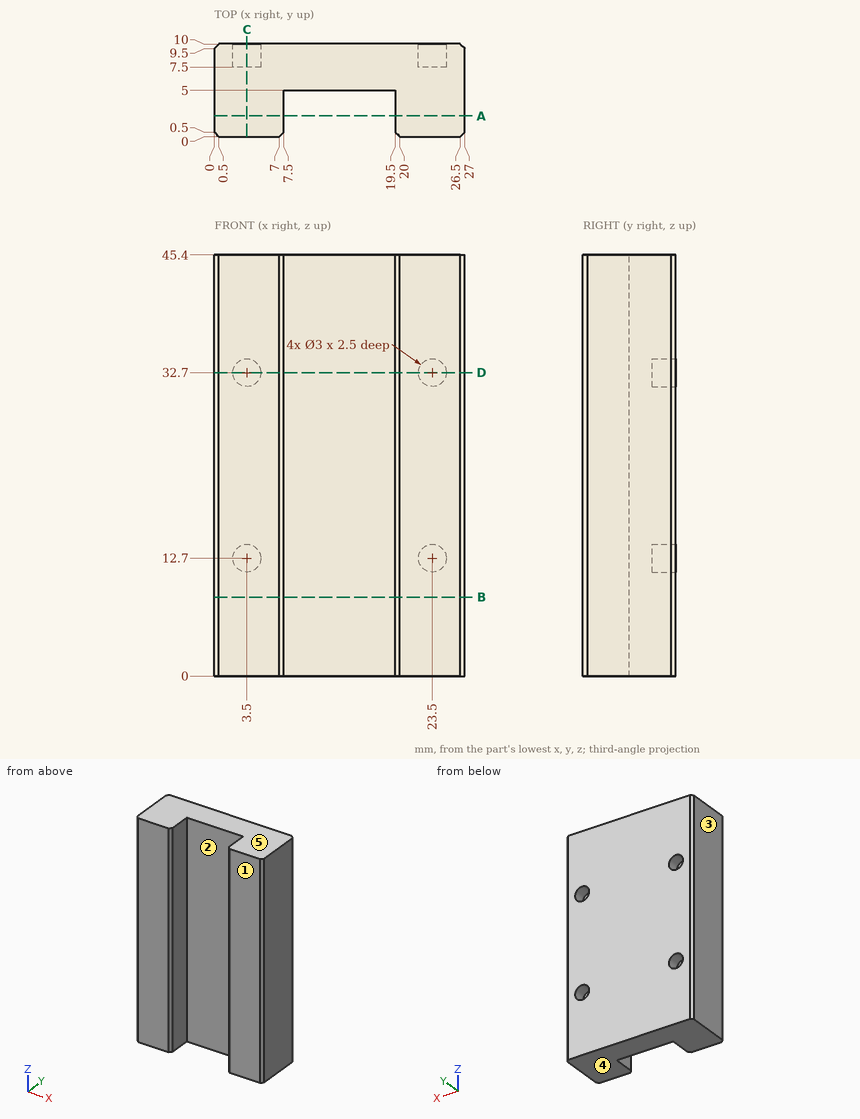
Here's the drawing with two shaded views (mm, measured from the low corner). I have some questions. A direction names the side the tool comes from. Give positions to 0.01 mm unless a question says otherwise; leave off trailing zeros. Loops run counter-clockwise (first coordinate to the right, second up) from the corner with the lowest first, then second, coordinate; pieces in that order, holes last. Notation, with made-up numbers: (41.5, 39) -> (65.5, 39) arc R17 cw to (65.5, 62) -> close; hole circle Ø11 at (-39, 62). An arc over 180 degrees is marked (long way). Answer as a JSON object with one key per item and string values. Group by question number.
Item 1: Imagine slicing it at A-A on y = 2.25. Write out the boundary of the cut face in (x, z), then the cut area to 3 significant figures.
Item 2: I need wall thicknesses on L1, parallel to Z at x = 23.5, y = 8.3; L2, parallel to X at y = 8.1, z = 12.7; L3, parallel to X at y = 2.5, z = 40. Which ranges of each line are inside material? Lowest first, please.
Item 3: Imagine slicing it at D-D on z = 32.7. Write out the boundary of the cut face in (x, y), then the cut area to 3 significant figures.
Item 4: Thinking about a two-plate mould opening in Z: for the marked faces 3, 4 and 5, which applies, pulls with the +Z half, pulls with the -Z half, needs draft (parallel to the pull), parting line crosses it, or undercut?
Item 5: On a 3-axis mill with a long thin cutter (end or side, diameter ignored), from which of +Z, -Z, +X, -X, +Y, -Y can I reach the whole of each face in a straight line? I mean the marked faces 1 and 2. Say none if no direction works.
Item 6: Imagine slicing it at B-B on z = 8.5. Write out the boundary of the cut face in (x, y), then the cut area to 3 significant figures.
Item 7: Imagine slicing it at C-C on x = 3.5. Write out the boundary of the cut face in (y, z).
Item 8: Will these pins go through, and if not, where does the flat tip stop? pin 1 (1.5 mm diameter, centred on x = 17, z = 38.5, fed in from -Y); pin 2 (2.5 mm diameter, centred on x = 23.5, z = 12.7, fed in from +Y).
Answer list:
{
 "1": {"outline": "(0, 0) -> (7.5, 0) -> (7.5, 45.4) -> (0, 45.4) -> close; (19.5, 0) -> (27, 0) -> (27, 45.4) -> (19.5, 45.4) -> close", "area": "681 mm2"},
 "2": {"L1": "z = 0 to 11.2, 14.2 to 31.2, 34.2 to 45.4", "L2": "x = 0 to 2, 5 to 22, 25 to 27", "L3": "x = 0 to 7.5, 19.5 to 27"},
 "3": {"outline": "(0, 0.5) -> (0.5, 0) -> (7, 0) -> (7.5, 0.5) -> (7.5, 5) -> (19.5, 5) -> (19.5, 0.5) -> (20, 0) -> (26.5, 0) -> (27, 0.5) -> (27, 9.5) -> (26.5, 10) -> (25, 10) -> (25, 7.5) -> (22, 7.5) -> (22, 10) -> (5, 10) -> (5, 7.5) -> (2, 7.5) -> (2, 10) -> (0.5, 10) -> (0, 9.5) -> close", "area": "194 mm2"},
 "4": {"face 3": "needs draft", "face 4": "pulls with the -Z half", "face 5": "pulls with the +Z half"},
 "5": {"face 1": "+Z, -Z, +X, -X, -Y", "face 2": "+Z, -Z, -Y"},
 "6": {"outline": "(0, 0.5) -> (0.5, 0) -> (7, 0) -> (7.5, 0.5) -> (7.5, 5) -> (19.5, 5) -> (19.5, 0.5) -> (20, 0) -> (26.5, 0) -> (27, 0.5) -> (27, 9.5) -> (26.5, 10) -> (0.5, 10) -> (0, 9.5) -> close", "area": "209 mm2"},
 "7": {"outline": "(0, 0) -> (10, 0) -> (10, 11.2) -> (7.5, 11.2) -> (7.5, 14.2) -> (10, 14.2) -> (10, 31.2) -> (7.5, 31.2) -> (7.5, 34.2) -> (10, 34.2) -> (10, 45.4) -> (0, 45.4) -> close"},
 "8": {"pin 1": "stops at y = 5", "pin 2": "stops at y = 7.5"}
}
